Can you work these out from the drawing? Everything is in mm from the part's minimum corner. A direction names the side the tool comes from. Give positions to 0.01 mm unless a question says otherwise; leave off trailing zeros. Order: outer loops, then holes, each group sorted by start corner. A loop starts at its lowest first (then second) coordinate and runs counter-clockwise, first axis right, second up. Notation, with made-up numbers: (14.25, 72) -> (57.25, 72) arc R16 ccw to (57.25, 91) -> close; hole circle Ø4 at (-22, 20). An arc over 180 degrees is marked (long way). One line per item, written item: value.
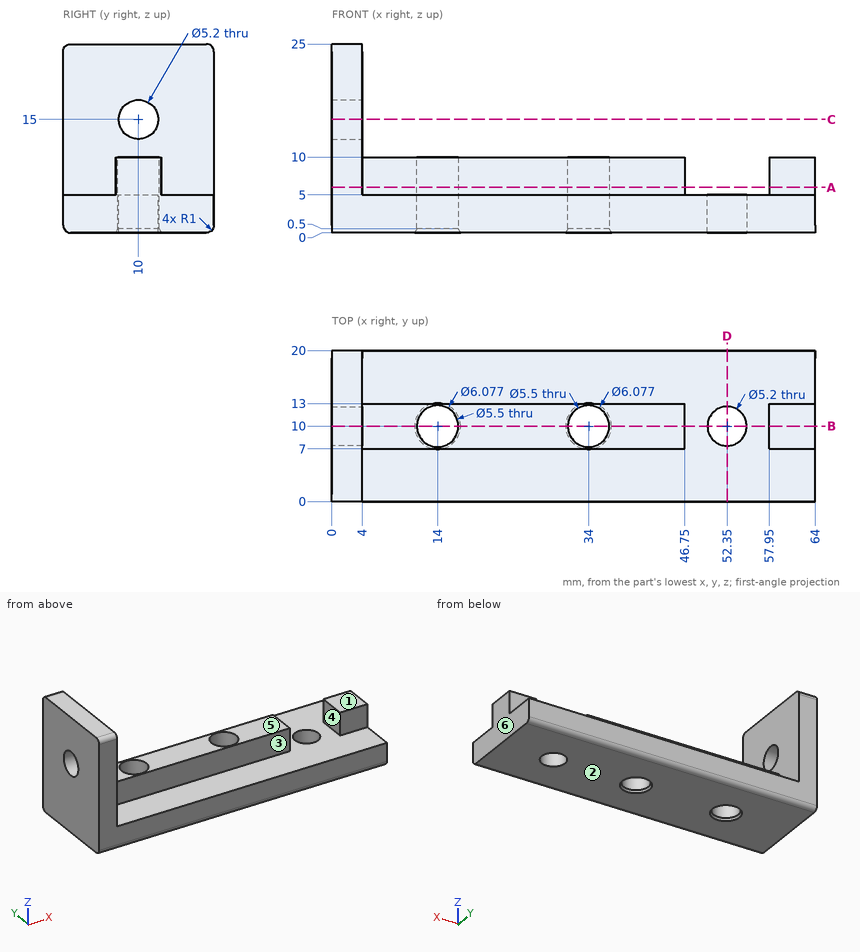
1) If I drill on line 1 along Z through (x, y) = (2.3, 10); line 2 along Y through (x, z) = (52.35, 3.2); line 3 along Z through (x, y) = (20, 1.5), over which ranges is the centre line in solid material (lowest first)?
Answer below:
line 1: z = 0 to 12.4, 17.6 to 25
line 2: y = 0 to 7.4, 12.6 to 20
line 3: z = 0 to 5
2) Suppose I cut it at B-B, the plane y = 10. State how many separate pieces and enclosed holes the cut face has, then the cut area to 3 significant figures.
Answer below:
separate pieces: 5
enclosed holes: 0
area: 487 mm2
3) Suppose I cut it at D-D, the plane x = 52.35. Write out the boundary of the cut face in (y, z).
Answer below:
outline: (0, 1) arc R1 ccw to (1, 0) -> (7.4, 0) -> (7.4, 5) -> (0, 5) -> close; (12.6, 0) -> (19, 0) arc R1 ccw to (20, 1) -> (20, 5) -> (12.6, 5) -> close
4) Suppose I cut it at A-A, the plane z = 6. Write out the boundary of the cut face in (x, y).
Answer below:
outline: (0, 0) -> (4, 0) -> (4, 7) -> (46.75, 7) -> (46.75, 13) -> (4, 13) -> (4, 20) -> (0, 20) -> close; (57.95, 7) -> (64, 7) -> (64, 13) -> (57.95, 13) -> close; hole circle Ø5.5 at (14, 10); hole circle Ø5.5 at (34, 10)
5) For P1, Ø3, axis at y = 13.5, z = 12.5, coming from the +X side; P2, Ø2.5, axis at x = 61, z = 7.5, coming from the -Y side; P3, Ø1.8, axis at x = 61.5, y = 9, coming from the +Z side, each with a flat end and sliding along its axis, tell me the tip position at first contact or that it passes through.
Answer below:
P1: stops at x = 4
P2: stops at y = 7
P3: stops at z = 10
6) For the marked faces 1, 2 and 3, which set-ups out of +Z, -Z, +X, -X, +Y, -Y let a thin tool reach every point of the face, with its end or its side?
Answer below:
face 1: +Z, +X, +Y, -Y
face 2: -Z, +X, -X, +Y, -Y
face 3: +Z, +X, -Y
7) We'd pull the mould along X, two halves only. Please class the marked faces 4, 5 and 6: +X half, -X half, draft (parallel to the pull), parting line (faces both ways), or undercut.
Answer below:
face 4: undercut
face 5: draft
face 6: +X half
8) Suppose I cut it at C-C, the plane z = 15. Write out the boundary of the cut face in (x, y).
Answer below:
outline: (0, 0) -> (4, 0) -> (4, 7.4) -> (0, 7.4) -> close; (0, 12.6) -> (4, 12.6) -> (4, 20) -> (0, 20) -> close
